Could you check a few things on this model? Use its own coordinates, in mm. Give positions to 0.01 mm unless a question says otherwise; leave off trailing zeros. Order: outer loops, then holes, each group sorted by start corner. A loop starts at its lowest first (then second) coordinate and runs counter-clockwise, first axis right, second up. Notation, with made-up numbers: M -13,-2.5 L -2,-2.5 A23 cw -2,23.5 Z; hole C -10.5,58.25 d4. An arc over 180 degrees is marked long. Use a Markdown table: item, result. Add a question column.
Item 1: Suppose I cut it at A-A on z = 0. Write out the boundary of the cut face in (x, y) (3 decimals), plus the area to 3 significant figures.
Item 2: If I drill on L1, parallel to Z at x = -8, y = -0.95; L2, parallel to X at y = -1.6, z = -14.5; L3, parallel to X at y = -2.45, z = 15, over which ranges is the centre line in solid material (lowest first)? Write a range as from..to.
Item 3: I'm going to push a flat-ended pin straight in: pin 1 Ø3 at (x, z) = (-157.63, -6.91) entering from -Y. Where does the tip first touch, or does it pass through?
Item 4: Suppose I cut it at C-C on z = 32. Write out the boundary of the cut face in (x, y) (3 decimals).
Item 5: Suppose I cut it at B-B on y = -1.5. Count the separate pieces of the cut face and the enclosed holes in it, plus the area to 3 significant figures.
from build123d import *

# Parameters (mm, degrees)
F0_R     = 2.25
F0_R_2   = 1.778
F0_R_3   = 4.7625
F0_R_4   = 19.05
F1_DEPTH = 3.175


with BuildPart() as f1:
    # F0 (on Front) → F1 (new body)
    with BuildSketch(Plane.XZ):
        with BuildLine():
            ThreePointArc((177.8, 12.7), (170.360512, 30.660512), (152.4, 38.1))
            Line((152.4, 38.1), (-152.4, 38.1))
            ThreePointArc((-152.4, 38.1), (-170.360512, 30.660512), (-177.8, 12.7))
            Line((-177.8, 12.7), (-177.8, -12.7))
            ThreePointArc((-177.8, -12.7), (-170.360512, -30.660512), (-152.4, -38.1))
            Line((-152.4, -38.1), (152.4, -38.1))
            ThreePointArc((152.4, -38.1), (170.360512, -30.660512), (177.8, -12.7))
            Line((177.8, -12.7), (177.8, 12.7))
        make_face()
        with Locations((-86.5112, -23.57)):
            Circle(F0_R, mode=Mode.SUBTRACT)
        with Locations((-39.3712, -23.57)):
            Circle(F0_R, mode=Mode.SUBTRACT)
        with Locations((-171.45, -6.9088)):
            Circle(F0_R_2, mode=Mode.SUBTRACT)
        with Locations((-157.6324, -6.9088)):
            Circle(F0_R_2, mode=Mode.SUBTRACT)
        with Locations((144.5006, -13.4747)):
            Circle(F0_R_2, mode=Mode.SUBTRACT)
        with Locations((171.45, -13.4747)):
            Circle(F0_R_2, mode=Mode.SUBTRACT)
        with Locations((-164.5412, 0)):
            Circle(F0_R_3, mode=Mode.SUBTRACT)
        with Locations((-171.45, 6.9088)):
            Circle(F0_R_2, mode=Mode.SUBTRACT)
        with Locations((-157.6324, 6.9088)):
            Circle(F0_R_2, mode=Mode.SUBTRACT)
        with Locations((-62.9412, 0)):
            Circle(F0_R_4, mode=Mode.SUBTRACT)
        with BuildLine():
            Line((-3.72745, 21.43125), (-3.72745, -21.43125))
            ThreePointArc((-3.72745, -21.43125), (-4.88987, -24.23758), (-7.6962, -25.4))
            ThreePointArc((-7.6962, -25.4), (-10.50253, -24.23758), (-11.66495, -21.43125))
            Line((-11.66495, -21.43125), (-11.66495, 21.43125))
            ThreePointArc((-11.66495, 21.43125), (-10.50253, 24.23758), (-7.6962, 25.4))
            ThreePointArc((-7.6962, 25.4), (-4.88987, 24.23758), (-3.72745, 21.43125))
        make_face(mode=Mode.SUBTRACT)
        with Locations((-86.5112, 23.57)):
            Circle(F0_R, mode=Mode.SUBTRACT)
        with Locations((-39.3712, 23.57)):
            Circle(F0_R, mode=Mode.SUBTRACT)
        with Locations((47.4853, 0)):
            Circle(F0_R_3, mode=Mode.SUBTRACT)
        with BuildLine():
            Line((106.69905, 21.43125), (106.69905, -21.43125))
            ThreePointArc((106.69905, -21.43125), (105.53663, -24.23758), (102.7303, -25.4))
            ThreePointArc((102.7303, -25.4), (99.92397, -24.23758), (98.76155, -21.43125))
            Line((98.76155, -21.43125), (98.76155, 21.43125))
            ThreePointArc((98.76155, 21.43125), (99.92397, 24.23758), (102.7303, 25.4))
            ThreePointArc((102.7303, 25.4), (105.53663, 24.23758), (106.69905, 21.43125))
        make_face(mode=Mode.SUBTRACT)
        with Locations((157.9753, 0)):
            Circle(F0_R_3, mode=Mode.SUBTRACT)
        with Locations((144.5006, 13.4747)):
            Circle(F0_R_2, mode=Mode.SUBTRACT)
        with Locations((171.45, 13.4747)):
            Circle(F0_R_2, mode=Mode.SUBTRACT)
    extrude(amount=F1_DEPTH)


solid = f1.part
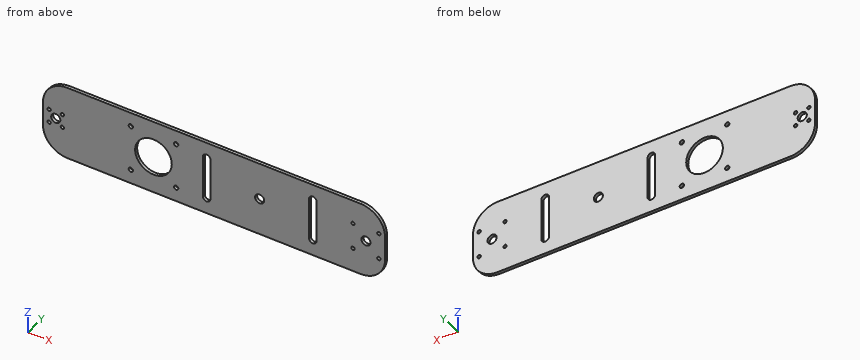
Findings below:
| question | item | result |
|---|---|---|
| 1 | outline | M -177.8,-3.175 L -169.304,-3.175 L -169.304,0 L -177.8,0 Z; M -159.779,-3.175 L -81.991,-3.175 L -81.991,0 L -159.779,0 Z; M -43.891,-3.175 L -11.665,-3.175 L -11.665,0 L -43.891,0 Z; M -3.727,-3.175 L 42.723,-3.175 L 42.723,0 L -3.727,0 Z; M 52.248,-3.175 L 98.762,-3.175 L 98.762,0 L 52.248,0 Z; M 106.699,-3.175 L 153.213,-3.175 L 153.213,0 L 106.699,0 Z; M 162.738,-3.175 L 177.8,-3.175 L 177.8,0 L 162.738,0 Z |
| 1 | area | 867 mm^2 |
| 2 | L1 | z = -38.1..-25.39, 25.39..38.1 |
| 2 | L2 | x = -177.74..-75.3, -50.59..-11.66, -3.73..98.76, 106.7..143.05, 145.95..170, 172.9..177.74 |
| 2 | L3 | x = -177.7..-74.68, -51.2..-11.66, -3.73..98.76, 106.7..143.59, 145.41..170.54, 172.36..177.7 |
| 3 | pin 1 | passes through |
| 4 | outline | M -168.913,-3.175 L 168.913,-3.175 L 168.913,0 L -168.913,0 Z |
| 5 | separate pieces | 1 |
| 5 | enclosed holes | 18 |
| 5 | area | 24,300 mm^2 |
